Check sheet for the modelled part. Datum: model origin and axes. Units: mm. A direction names the side the tool comes from. Give positions to 0.01 mm unless a question says otherwise; leave off trailing zeros. Write each loop counter-clockwise with the first axis right and the second up, starting at its lowest first coordinate (ties: lowest second). Pieces come first, ordered by that corner, then holes. Notation, with made-up numbers: (-2, 84.25) -> (55, 84.25) arc R18 ccw to (55, 105.25) -> close; hole circle Ø2 at (32, 43). An arc over 180 degrees is marked (long way). Answer as a JSON object with one key per item and string values.
from build123d import *

# Parameters (mm, degrees)
SKETCH3_W           = 150
SKETCH3_H           = 150
BOSS_EXTRUDE1_DEPTH = 30
SHELL1_T            = -5
CUT_EXTRUDE1_DEPTH  = 20
FILLET2_R           = 2


with BuildPart() as part:
    # Sketch3 → Boss-Extrude1 (new body)
    with BuildSketch(Plane(origin=(0, 0, 0), x_dir=(1, 0, 0), z_dir=(0, 1, 0))):
        with Locations((75, 75)):
            Rectangle(SKETCH3_W, SKETCH3_H)
    extrude(amount=BOSS_EXTRUDE1_DEPTH)

    # Shell1
    shell1_openings = [part.faces().sort_by_distance(p)[0] for p in [
        (75, 30, -75),
    ]]
    offset(amount=SHELL1_T, openings=shell1_openings, kind=Kind.INTERSECTION)

    # Sketch5 → Cut-Extrude1 (cut)
    with BuildSketch(Plane(origin=(0, 30, 0), x_dir=(1, 0, 0), z_dir=(0, 1, 0))):
        Polygon((1.35, 148.65), (36.55, 148.65), (36.55, 146.35), (3.65, 146.35), (3.65, 113.45), (1.35, 113.45), align=None)
        Polygon((148.65, 113.45), (148.65, 148.65), (113.45, 148.65), (113.45, 146.35), (146.35, 146.35), (146.35, 113.45), align=None)
        Polygon((148.65, 1.35), (113.45, 1.35), (113.45, 3.65), (146.35, 3.65), (146.35, 36.55), (148.65, 36.55), align=None)
        Polygon((1.35, 36.55), (1.35, 1.35), (36.55, 1.35), (36.55, 3.65), (3.65, 3.65), (3.65, 36.55), align=None)
    extrude(amount=-CUT_EXTRUDE1_DEPTH, mode=Mode.SUBTRACT)

    # Fillet2
    fillet2_edges = [part.edges().sort_by_distance(p)[0] for p in [
        (0, 15, -150),
        (150, 15, -150),
        (150, 15, 0),
        (0, 15, 0),
    ]]
    fillet(fillet2_edges, radius=FILLET2_R)


solid = part.part
1. Sectioned sample at C-C, the plane y = 24.25. State how many separate pieces and enclosed holes the cut face has, plus the area to 3 significant figures.
Determined:
{"separate pieces": "1", "enclosed holes": "5", "area": "2,270 mm^2"}
2. Access from +Z, -Z, +X, -X, +Y, -Y to the whole of each face (thin tool, end or side, straight path). Record for faces 1 (the face through (1.35, 20, -131)), 2 (the face through (74, 15, -150)).
Determined:
{"face 1": "+Y", "face 2": "-Z, +X, -X, +Y, -Y"}
3. Sectioned sample at D-D, the plane z = -73. Enter the section's corners in (x, y), plus the area to 3 significant figures.
Determined:
{"outline": "(0, 0) -> (150, 0) -> (150, 30) -> (145, 30) -> (145, 5) -> (5, 5) -> (5, 30) -> (0, 30) -> close", "area": "1,000 mm^2"}
4. Sectioned sample at A-A, the plane x = 137. Enter the section's corners in (y, z).
Determined:
{"outline": "(0, -150) -> (30, -150) -> (30, -148.65) -> (10, -148.65) -> (10, -146.35) -> (30, -146.35) -> (30, -145) -> (5, -145) -> (5, -5) -> (30, -5) -> (30, -3.65) -> (10, -3.65) -> (10, -1.35) -> (30, -1.35) -> (30, 0) -> (0, 0) -> close"}
5. Go/stop test with a flat-tipped pin: P1, Ø4, axis at x = 128.5, z = -93.5, coming from the +Y side. Record where the tip stops, or that it passes through.
Determined:
{"P1": "y = 5"}
6. Scan lines: L1, parallel to X at y = 27.5, z = -123; L2, parallel to Z at x = 117, y = 5.25; L3, parallel to Z at x = 12, y = 26.25. Record each from-to range of solid material in increasing order. Write a range as [from, to].
Determined:
{"L1": "[0, 1.35], [3.65, 5], [145, 146.35], [148.65, 150]", "L2": "[-150, -145], [-5, 0]", "L3": "[-150, -148.65], [-146.35, -145], [-5, -3.65], [-1.35, 0]"}
7. Sectioned sample at B-B, the plane z = -123.5. Enter the section's corners in (x, y).
Determined:
{"outline": "(0, 0) -> (150, 0) -> (150, 30) -> (148.65, 30) -> (148.65, 10) -> (146.35, 10) -> (146.35, 30) -> (145, 30) -> (145, 5) -> (5, 5) -> (5, 30) -> (3.65, 30) -> (3.65, 10) -> (1.35, 10) -> (1.35, 30) -> (0, 30) -> close"}
